from build123d import *

# Parameters (mm, degrees)
SKETCH1_W                                = 45
SKETCH1_H                                = 30
BOSS_EXTRUDE1_DEPTH                      = 22
SKETCH3_W                                = 20
SKETCH3_H                                = 20
CUT_EXTRUDE1_DEPTH                       = 16
CBORE_FOR_M3_PAN_HEAD_SCREW4_D           = 3.4
CBORE_FOR_M3_PAN_HEAD_SCREW4_CBORE_D     = 7
CBORE_FOR_M3_PAN_HEAD_SCREW4_CBORE_DEPTH = 19.4


with BuildPart() as part:
    # Sketch1 → Boss-Extrude1 (new body)
    with BuildSketch(Plane(origin=(0, 0, 0), x_dir=(0, 0, -1), z_dir=(1, 0, 0))):
        with Locations((22.5, 15)):
            Rectangle(SKETCH1_W, SKETCH1_H)
    extrude(amount=BOSS_EXTRUDE1_DEPTH)

    # Sketch3 → Cut-Extrude1 (cut)
    with BuildSketch(Plane(origin=(22, 0, 0), x_dir=(0, 0, -1), z_dir=(1, 0, 0))):
        with Locations((22.5, 15)):
            Rectangle(SKETCH3_W, SKETCH3_H)
    extrude(amount=-CUT_EXTRUDE1_DEPTH, mode=Mode.SUBTRACT)

    # CBORE for M3 Pan Head Screw4 (through all)
    with Locations(Plane(origin=(22, 0, 0), x_dir=(0, 0, -1), z_dir=(1, 0, 0))):
        with Locations((12.5, 25), (32.5, 25), (32.5, 5), (12.5, 5)):
            CounterBoreHole(CBORE_FOR_M3_PAN_HEAD_SCREW4_D / 2, CBORE_FOR_M3_PAN_HEAD_SCREW4_CBORE_D / 2, CBORE_FOR_M3_PAN_HEAD_SCREW4_CBORE_DEPTH)


solid = part.part
Design review of the part built by this model. Coordinates are the model's own, in mm. A direction names the side the tool comes from. Round coordinates to 2 decimals unless told otherwise and drop trailing zeros. Order: outer loops, then holes, each group sorted by start corner. A loop starts at its lowest first (then second) coordinate and runs counter-clockwise, first axis right, second up. Notation, with made-up numbers: M 62,49.5 L 74,49.5 A18 cw 74,56.5 Z; hole C 41,23 d10. An arc over 180 degrees is marked long. Answer as CSV lines item,"result". Start each with the question number.
1) Add section D-D (z = -25.5). Give the boundary of the cut face in (x, y), then the cut area to 3 significant figures.
2) For pin 1 Ø6.5 at (y, z) = (25, -12.5) entering from +X; pin 2 Ø1.5 at (y, z) = (14, -28) entering from +X, all flat-tipped, find the tip position at first contact; note any pin that passes through.
3) The part is to be moulded in two halves that separate along Z. For faces 1 (the face through (11, 30, -22)), 2 (the face through (14, 15, -12.5)), 3 (the face through (11, 15, -45)), 4 (the face through (14, 15, -32.5)), say which applies: +Z half, -Z half, draft (parallel to the pull), parting line (faces both ways), or undercut.
4) Add section A-A (x = 15.75). Give the boundary of the cut face in (y, z), then the cut area to 3 significant figures.
5) Tool access review of faces 5 (the face through (2.6, 3, -12)), 6 (the face through (22, 25.2, -22.2)): name each direction out of +Z, -Z, +X, -X, +Y, -Y from which nothing blocks a thin tool from reaching the whole face with its end or side.
6) Add section C-C (y = 10.25). Give the boundary of the cut face in (x, z).
7) Wall thickness on line 1 along Z through (x, y) = (10.5, 25.25); line 2 along Z through (x, y) = (19.75, 15.5); line 3 along Y through (x, z) = (21, -19): over which ranges is each line inside the solid? List them lowest first. Write a range as [from, to].
8) Add section B-B (z = -33). Give the boundary of the cut face in (x, y), then the cut area to 3 significant figures.
Resolved:
1,outline,"M 0,0 L 22,0 L 22,5 L 6,5 L 6,25 L 22,25 L 22,30 L 0,30 Z"
1,area,"340 mm^2"
2,pin 1,"x = 2.6"
2,pin 2,"x = 6"
3,face 1,"draft"
3,face 2,"undercut"
3,face 3,"-Z half"
3,face 4,"undercut"
4,outline,"M 0,-45 L 30,-45 L 30,0 L 0,0 Z; hole M 5,-29 A3.5 ccw long 8.5,-32.5 L 21.5,-32.5 A3.5 ccw long 25,-29 L 25,-16 A3.5 ccw long 21.5,-12.5 L 8.5,-12.5 A3.5 ccw long 5,-16 Z"
4,area,"835 mm^2"
5,face 5,"+X"
5,face 6,"+Z, -Z, +X, +Y, -Y"
6,outline,"M 0,-45 L 22,-45 L 22,-32.5 L 6,-32.5 L 6,-12.5 L 22,-12.5 L 22,0 L 0,0 Z"
7,line 1,"[-45, -35.99], [-29.01, -15.99], [-9.01, 0]"
7,line 2,"[-45, -32.5], [-12.5, 0]"
7,line 3,"[0, 5], [25, 30]"
8,outline,"M 0,0 L 22,0 L 22,1.54 L 2.6,1.54 L 2.6,3.38 L 0,3.38 Z; M 0,6.62 L 2.6,6.62 L 2.6,8.46 L 22,8.46 L 22,21.54 L 2.6,21.54 L 2.6,23.38 L 0,23.38 Z; M 0,26.62 L 2.6,26.62 L 2.6,28.46 L 22,28.46 L 22,30 L 0,30 Z"
8,area,"374 mm^2"
